from build123d import *

# Parameters (mm, degrees)
SKETCH1_R           = 5
BOSS_EXTRUDE1_DEPTH = 45
SKETCH2_R           = 19
SKETCH2_R_2         = 5
BOSS_EXTRUDE2_DEPTH = 1.5
SKETCH3_R           = 2.5
CUT_EXTRUDE1_DEPTH  = 61.128861622
SKETCH4_R           = 2.5
CUT_EXTRUDE2_DEPTH  = 40.1
FILLET1_R           = 3.5


with BuildPart() as part:
    # Sketch1 → Boss-Extrude1 (new body)
    with BuildSketch(Plane.XY):
        with BuildLine():
            Line((-24.7, -28.2), (24.7, -28.2))
            ThreePointArc((24.7, -28.2), (27.174873734, -27.174873734), (28.2, -24.7))
            Line((28.2, -24.7), (28.2, 24.7))
            ThreePointArc((28.2, 24.7), (27.174873734, 27.174873734), (24.7, 28.2))
            Line((24.7, 28.2), (-24.7, 28.2))
            ThreePointArc((-24.7, 28.2), (-27.174873734, 27.174873734), (-28.2, 24.7))
            Line((-28.2, 24.7), (-28.2, -24.7))
            ThreePointArc((-28.2, -24.7), (-27.174873734, -27.174873734), (-24.7, -28.2))
        make_face()
        with Locations(Location((0, 0, 0), (0, 0, 180))):
            Circle(SKETCH1_R, mode=Mode.SUBTRACT)
    extrude(amount=BOSS_EXTRUDE1_DEPTH)

    # Sketch2 → Boss-Extrude2 (add)
    with BuildSketch(Plane.XY.offset(45)):
        Circle(SKETCH2_R)
        with Locations(Location((0, 0, 0), (0, 0, 180))):
            Circle(SKETCH2_R_2, mode=Mode.SUBTRACT)
    extrude(amount=BOSS_EXTRUDE2_DEPTH)

    # Sketch3 → Cut-Extrude1 (cut, through all)
    with BuildSketch(Plane.XY.offset(45)):
        with Locations((-23.55, 23.55)):
            Circle(SKETCH3_R)
        with Locations((23.55, 23.55)):
            Circle(SKETCH3_R)
        with Locations((23.55, -23.55)):
            Circle(SKETCH3_R)
        with Locations((-23.55, -23.55)):
            Circle(SKETCH3_R)
    extrude(amount=-CUT_EXTRUDE1_DEPTH, mode=Mode.SUBTRACT)

    # Sketch4 → Cut-Extrude2 (cut)
    # profile 1 of 4: a face of its own
    with BuildSketch(Plane(origin=(0, 0, 0), x_dir=(-1, 0, 0), z_dir=(0, 0, -1))):
        with BuildLine():
            ThreePointArc((-28.2, 17.2), (-20.421825407, 20.421825407), (-17.2, 28.2))
            Line((-17.2, 28.2), (-24.7, 28.2))
            ThreePointArc((-24.7, 28.2), (-27.174873734, 27.174873734), (-28.2, 24.7))
            Line((-28.2, 24.7), (-28.2, 17.2))
        make_face()
        with Locations(Location((-23.55, 23.55, 0), (0, 0, 180))):
            Circle(SKETCH4_R, mode=Mode.SUBTRACT)
    # profile 2 of 4: a face of its own
    with BuildSketch(Plane(origin=(0, 0, 0), x_dir=(-1, 0, 0), z_dir=(0, 0, -1))):
        with BuildLine():
            Line((-24.7, -28.2), (-17.2, -28.2))
            ThreePointArc((-17.2, -28.2), (-20.421825407, -20.421825407), (-28.2, -17.2))
            Line((-28.2, -17.2), (-28.2, -24.7))
            ThreePointArc((-28.2, -24.7), (-27.174873734, -27.174873734), (-24.7, -28.2))
        make_face()
        with Locations(Location((-23.55, -23.55, 0), (0, 0, 180))):
            Circle(SKETCH4_R, mode=Mode.SUBTRACT)
    # profile 3 of 4: a face of its own
    with BuildSketch(Plane(origin=(0, 0, 0), x_dir=(-1, 0, 0), z_dir=(0, 0, -1))):
        with BuildLine():
            Line((28.2, -24.7), (28.2, -17.2))
            ThreePointArc((28.2, -17.2), (20.421825407, -20.421825407), (17.2, -28.2))
            Line((17.2, -28.2), (24.7, -28.2))
            ThreePointArc((24.7, -28.2), (27.174873734, -27.174873734), (28.2, -24.7))
        make_face()
        with Locations(Location((23.55, -23.55, 0), (0, 0, 180))):
            Circle(SKETCH4_R, mode=Mode.SUBTRACT)
    # profile 4 of 4: a face of its own
    with BuildSketch(Plane(origin=(0, 0, 0), x_dir=(-1, 0, 0), z_dir=(0, 0, -1))):
        with BuildLine():
            ThreePointArc((17.2, 28.2), (20.421825407, 20.421825407), (28.2, 17.2))
            Line((28.2, 17.2), (28.2, 24.7))
            ThreePointArc((28.2, 24.7), (27.174873734, 27.174873734), (24.7, 28.2))
            Line((24.7, 28.2), (17.2, 28.2))
        make_face()
        with Locations(Location((23.55, 23.55, 0), (0, 0, 180))):
            Circle(SKETCH4_R, mode=Mode.SUBTRACT)
    extrude(amount=-CUT_EXTRUDE2_DEPTH, mode=Mode.SUBTRACT)

    # Fillet1
    fillet1_edges = [part.edges().sort_by_distance(p)[0] for p in [
        (-17.2, 28.2, 20.05),
        (-28.2, 17.2, 20.05),
        (-17.2, -28.2, 20.05),
        (-28.2, -17.2, 20.05),
        (28.2, -17.2, 20.05),
        (17.2, -28.2, 20.05),
        (28.2, 17.2, 20.05),
        (17.2, 28.2, 20.05),
    ]]
    fillet(fillet1_edges, radius=FILLET1_R)


solid = part.part
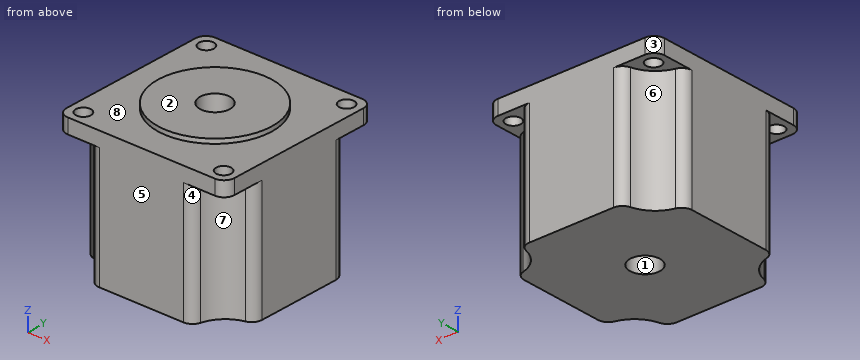
Read the model definition and answer for the solid it produces. Units are mm, in the model's axes. Face numbers are marked on the shaded views. A direction names the side the tool comes from. Give positions to 0.01 mm unless a question says otherwise; leave off trailing zeros. Write each loop counter-clockwise with the first axis right and the second up, starting at its lowest first coordinate (ties: lowest second). Pieces come first, ordered by that corner, then holes. Notation, with made-up numbers: M 74.25,14.25 L 79.25,14.25 A23 ccw 79.25,23.25 Z; hole C -20,66.5 d6. An arc over 180 degrees is marked long. One line per item, written item: value. Start each with the question number.
(1) Find section D-D (z = 32). Determine the outline of the cut face in (x, y).
(2) Flat-ended cylindrical pins translate along their axes: pin 1 Ø11.5 at (x, y) = (-24.5, -22.5) entering from -Z; pin 2 Ø6 at (x, y) = (-23.55, -23.55) entering from +Z; pin 3 Ø4 at (x, y) = (-22, 22.5) entering from -Z; pin 4 Ø6 at (y, z) = (-17.5, 12) entering from +X. Find the tip coordinate at first contact, or state that the pin passes through.
(3) Find section A-A (x = 0). Determine the outline of the cut face in (y, z).
(4) Determine the mould class of the marked faces 1, 2, 3 and 4 for opening direction X: pulls with the +X half, pulls with the -X half, needs draft (parallel to the pull), parting line crosses it, or undercut.
(5) Find the intervals of material crossed by line 1 (Y direction, x = -23.55, z = 43.25); line 2 (Z direction, x = -17.5, y = 19), in increasing order.
(6) A tool of negligible diameter and unlimited length cuts with its end or side. For the marked faces 5, 6, 7 and 8, from which of +Z, -Z, +X, -X, +Y, -Y can it reach the whole face along a straight path? Write none if from no direction.
(7) Find section B-B (y = 23.55). Determine the outline of the cut face in (x, z).
Results below:
1. outline: M -28.2,-14.13 A3.5 ccw -25.54,-17.53 A11 cw -17.53,-25.54 A3.5 ccw -14.13,-28.2 L 14.13,-28.2 A3.5 ccw 17.53,-25.54 A11 cw 25.54,-17.53 A3.5 ccw 28.2,-14.13 L 28.2,14.13 A3.5 ccw 25.54,17.53 A11 cw 17.53,25.54 A3.5 ccw 14.13,28.2 L -14.13,28.2 A3.5 ccw -17.53,25.54 A11 cw -25.54,17.53 A3.5 ccw -28.2,14.13 Z; hole C 0,0 d10
2. pin 1: stops at z = 0
2. pin 2: stops at z = 45
2. pin 3: stops at z = 40.1
2. pin 4: stops at x = 28.18
3. outline: M -28.2,0 L -5,0 L -5,46.5 L -19,46.5 L -19,45 L -28.2,45 Z; M 5,0 L 28.2,0 L 28.2,45 L 19,45 L 19,46.5 L 5,46.5 Z
4. face 1: undercut
4. face 2: needs draft
4. face 3: pulls with the -X half
4. face 4: pulls with the +X half
5. line 1: y = -28.2 to -26.05, -21.05 to 21.05, 26.05 to 28.2
5. line 2: z = 0 to 45
6. face 5: +Z, -Z, +X, -X, -Y
6. face 6: -Z, -X, +Y
6. face 7: -Z, +X, -Y
6. face 8: +Z
7. outline: M -28.2,40.1 L -26.05,40.1 L -26.05,45 L -28.2,45 Z; M -21.05,40.1 L -18.23,40.1 L -18.23,0 L 18.23,0 L 18.23,40.1 L 21.05,40.1 L 21.05,45 L -21.05,45 Z; M 26.05,40.1 L 28.2,40.1 L 28.2,45 L 26.05,45 Z
